```python
from build123d import *

# Parameters (mm, degrees)
SKETCH_2_W                      = 50
SKETCH_2_H                      = 50
EXTRUDE_1_DEPTH                 = 35
SKETCH_3_R                      = 20
CUT_EXTRUDE_1_DEPTH             = 20
HOLE_WIZARD_G1_16_1_D           = 6.6
HOLE_WIZARD_G1_16_1_DEPTH       = 20
HOLE_WIZARD_G1_16_1_CSINK_D     = 7.773
HOLE_WIZARD_G1_16_1_CSINK_ANGLE = 90
HOLE_WIZARD_G1_16_1_TIP         = 1.982840043
SKETCH_6_W                      = 35
SKETCH_6_H                      = 10
EXTRUDE_2_DEPTH                 = 30
SKETCH_7_W                      = 35
SKETCH_7_H                      = 10
EXTRUDE_3_DEPTH                 = 40
HOLE_WIZARD_G1_16_2_D           = 6.6
HOLE_WIZARD_G1_16_2_DEPTH       = 20
HOLE_WIZARD_G1_16_2_CSINK_D     = 7.773
HOLE_WIZARD_G1_16_2_CSINK_ANGLE = 90
HOLE_WIZARD_G1_16_2_TIP         = 1.982840043


with BuildPart() as part:
    # 草图2 → 凸台-拉伸1 (new body)
    with BuildSketch(Plane(origin=(0, 0, 0), x_dir=(0, 0, -1), z_dir=(1, 0, 0))):
        with Locations((25, -25)):
            Rectangle(SKETCH_2_W, SKETCH_2_H)
    extrude(amount=EXTRUDE_1_DEPTH)

    # 草图3 → 切除-拉伸1 (cut)
    with BuildSketch(Plane.ZY):
        with Locations((-25, -25)):
            Circle(SKETCH_3_R)
    extrude(amount=-CUT_EXTRUDE_1_DEPTH, mode=Mode.SUBTRACT)

    # G1/16 螺纹孔1
    with Locations(Plane(origin=(35, 0, 0), x_dir=(0, 0, -1), z_dir=(1, 0, 0))):
        with Locations((25, -25)):
            CounterSinkHole(HOLE_WIZARD_G1_16_1_D / 2, HOLE_WIZARD_G1_16_1_CSINK_D / 2, depth=HOLE_WIZARD_G1_16_1_DEPTH, counter_sink_angle=HOLE_WIZARD_G1_16_1_CSINK_ANGLE)
            with Locations((0, 0, -(HOLE_WIZARD_G1_16_1_DEPTH + HOLE_WIZARD_G1_16_1_TIP / 2))):  # 118° drill point
                Cone(0, HOLE_WIZARD_G1_16_1_D / 2, HOLE_WIZARD_G1_16_1_TIP, mode=Mode.SUBTRACT)

    # 草图6 → 凸台-拉伸2 (add)
    with BuildSketch(Plane(origin=(0, 0, -50), x_dir=(-1, 0, 0), z_dir=(0, 0, -1))):
        with Locations((-17.5, -5)):
            Rectangle(SKETCH_6_W, SKETCH_6_H)
    extrude(amount=EXTRUDE_2_DEPTH)

    # 草图7 → 凸台-拉伸3 (add)
    with BuildSketch(Plane(origin=(0, -10, 0), x_dir=(-1, 0, 0), z_dir=(0, -1, 0))):
        with Locations((-17.5, 75)):
            Rectangle(SKETCH_7_W, SKETCH_7_H)
    extrude(amount=EXTRUDE_3_DEPTH)

    # G1/16 螺纹孔2
    with Locations(Plane(origin=(0, 0, -80), x_dir=(-1, 0, 0), z_dir=(0, 0, -1))):
        with Locations((-17.5, -35)):
            CounterSinkHole(HOLE_WIZARD_G1_16_2_D / 2, HOLE_WIZARD_G1_16_2_CSINK_D / 2, depth=HOLE_WIZARD_G1_16_2_DEPTH, counter_sink_angle=HOLE_WIZARD_G1_16_2_CSINK_ANGLE)
            with Locations((0, 0, -(HOLE_WIZARD_G1_16_2_DEPTH + HOLE_WIZARD_G1_16_2_TIP / 2))):  # 118° drill point
                Cone(0, HOLE_WIZARD_G1_16_2_D / 2, HOLE_WIZARD_G1_16_2_TIP, mode=Mode.SUBTRACT)


solid = part.part
```
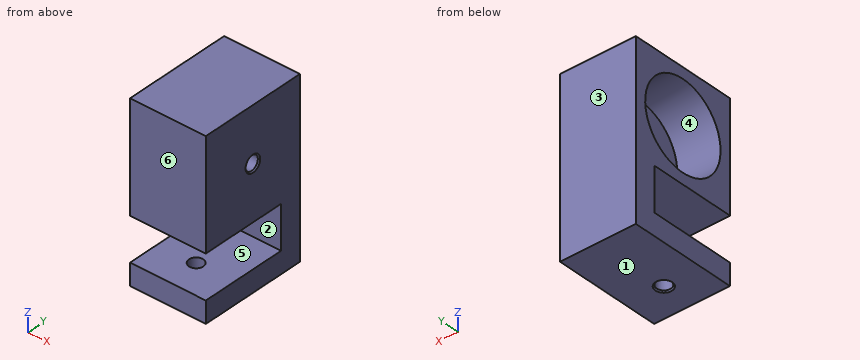
Check sheet for the modelled part. Datum: model origin and axes. Units: mm. Face numbers are marked on the shaded views. A direction names the side the tool comes from. Give positions to 0.01 mm unless a question says otherwise; leave off trailing zeros. Write each loop counter-clockwise with the first axis right and the second up, starting at its lowest first coordinate (ties: lowest second). Pieces come first, ordered by that corner, then holes. Notation, with made-up numbers: (11.25, 89.25) -> (68.25, 89.25) arc R22 cw to (68.25, 122.25) -> close; hole circle Ø6 at (53.25, 47.25). An arc over 180 degrees is marked (long way). Use CSV: the item, a comma, the result in double quotes. Start each with the question number.
Q1. Cross-section at C-C on z = -25. Enter the section's corners in (x, y).
Q2. Depth check by flat-ended pin: P1, Ø24, axis at y = -25, z = -25, coming from the -X side; P2, Ø6, axis at x = 17.5, y = -35, coming from the -Z side; P3, Ø10, axis at x = 12.5, z = -59, coming from the -Y side. Enter the tip coordinate at first touch or a pass-through.
Q3. Cross-section at A-A on x = 6.5. Enter the section's corners in (y, z), and give its area (3 significant figures).
Q4. Scan lines: line 1 along Z through (x, y) = (28.5, -25); line 2 along Z through (x, y) = (26, -19); line 3 along Z through (x, y) = (10, -21.5). Record each from-to range of solid material in increasing order.
Q5. Release check for a two-part mould opening along Z. For the marked faces 1, 2 and 3 record: +Z half, -Z half, draft (parallel to the pull), parting line (faces both ways), or undercut.
Q6. Tool access check on the marked faces 4, 5 and 6. Record the directions out of +Z, -Z, +X, -X, +Y, -Y that give a thin tool (end or side, any length) a straight path to the whole face; none if there is none.
Q7. Cross-section at D-D on y = -25. Enter the section's corners in (x, z), and give its area (3 significant figures).
Q8. Cross-section at B-B on x = 17.5. Enter the section's corners in (y, z), and give its area (3 significant figures).
Working result:
1,outline,"(0, -50) -> (35, -50) -> (35, -28.89) -> (34.41, -28.3) -> (20, -28.3) -> (20, -45) -> (0, -45) -> close; (0, -5) -> (20, -5) -> (20, -21.7) -> (34.41, -21.7) -> (35, -21.11) -> (35, 0) -> (0, 0) -> close"
2,P1,"stops at x = 20"
2,P2,"stops at z = -50"
2,P3,"stops at y = -10"
3,outline,"(-50, -80) -> (0, -80) -> (0, 0) -> (-50, 0) -> (-50, -50) -> (-10, -50) -> (-10, -70) -> (-50, -70) -> close; hole circle Ø40 at (-25, -25)"
3,area,"1,940 mm^2"
4,line 1,"z = -80 to -70, -50 to -28.3, -21.7 to 0"
4,line 2,"z = -80 to -70, -50 to 0"
4,line 3,"z = -80 to -70, -50 to -44.69, -5.31 to 0"
5,face 1,"-Z half"
5,face 2,"undercut"
5,face 3,"draft"
6,face 4,"-X"
6,face 5,"+X, -X, -Y"
6,face 6,"+Z, -Z, +X, -X, -Y"
7,outline,"(0, -80) -> (35, -80) -> (35, -70) -> (0, -70) -> close; (0, -50) -> (35, -50) -> (35, -28.89) -> (34.41, -28.3) -> (20, -28.3) -> (20, -45) -> (0, -45) -> close; (0, -5) -> (20, -5) -> (20, -21.7) -> (34.41, -21.7) -> (35, -21.11) -> (35, 0) -> (0, 0) -> close"
7,area,"1,200 mm^2"
8,outline,"(-50, -80) -> (-38.89, -80) -> (-38.3, -79.41) -> (-38.3, -70) -> (-50, -70) -> close; (-50, -50) -> (-10, -50) -> (-10, -70) -> (-31.7, -70) -> (-31.7, -79.41) -> (-31.11, -80) -> (0, -80) -> (0, 0) -> (-50, 0) -> close; hole circle Ø40 at (-25, -25)"
8,area,"1,880 mm^2"
